from build123d import *

# Parameters (mm, degrees)
SKETCH2_W      = 150
SKETCH2_H      = 70
EXTRUDE1_DEPTH = 20
SKETCH3_W      = 20.4
SKETCH3_H      = 20.4
EXTRUDE2_DEPTH = 20
SKETCH6_W      = 20.4
SKETCH6_H      = 20.4
EXTRUDE5_DEPTH = 20
EXTRUDE6_DEPTH = 20


with BuildPart() as part:
    # Sketch2 → Extrude1 (new body)
    with BuildSketch(Plane(origin=(0, 0, 0), x_dir=(1, 0, 0), z_dir=(0, 1, 0))):
        Rectangle(SKETCH2_W, SKETCH2_H)
    extrude(amount=EXTRUDE1_DEPTH)

    # Sketch3 → Extrude2 (cut)
    with BuildSketch(Plane(origin=(0, 20, 0), x_dir=(1, 0, 0), z_dir=(0, 1, 0))):
        with Locations((0, 12.2)):
            Rectangle(SKETCH3_W, SKETCH3_H)
    extrude(amount=-EXTRUDE2_DEPTH, mode=Mode.SUBTRACT)

    # Sketch6 → Extrude5 (cut)
    with BuildSketch(Plane(origin=(0, 20, 0), x_dir=(1, 0, 0), z_dir=(0, 1, 0))):
        with Locations((-57.5, 4.8)):
            Rectangle(SKETCH6_W, SKETCH6_H)
        with Locations((57.5, 4.8)):
            Rectangle(SKETCH6_W, SKETCH6_H)
    extrude(amount=-EXTRUDE5_DEPTH, mode=Mode.SUBTRACT)

    # Sketch7 → Extrude6 (cut)
    with BuildSketch(Plane(origin=(0, 20, 0), x_dir=(1, 0, 0), z_dir=(0, 1, 0))):
        Polygon((-70.635231965, -35), (-75, -32.48), (-75, -35), align=None)
        Polygon((-75, 35), (-70.635231965, 35), (-75, 32.48), align=None)
        Polygon((75, -35), (70.635231965, -35), (75, -32.48), align=None)
        Polygon((70.635231965, 35), (75, 32.48), (75, 35), align=None)
    extrude(amount=-EXTRUDE6_DEPTH, mode=Mode.SUBTRACT)


solid = part.part
CAD build for the part. Positions are in the model's coordinates, mm. A direction names the side the tool comes from. Give positions to 0.01 mm unless a question says otherwise; leave off trailing zeros. Write each loop counter-clockwise with the first axis right and the second up, starting at its lowest first coordinate (ties: lowest second). Pieces come first, ordered by that corner, then holes. Notation, with made-up numbers: (43, -22.75) - (61, -22.75) arc R19 ccw to (61, -1.75) - close; hole circle Ø1 at (46, 1.25). An arc over 180 degrees is marked (long way). Answer as CSV lines item,"result".
Q1. Drill centre lines: line 1 (X direction, y = 18, z = -6); line 2 (Z direction, x = 58.5, y = 5.75); line 3 (Z direction, x = 7, y = 13.25). Where is each one in solid material? Low to high. Write a range as from..to.
Result set:
line 1,"-75..-67.7, -47.3..-10.2, 10.2..47.3, 67.7..75"
line 2,"-35..-15, 5.4..35"
line 3,"-35..-22.4, -2..35"
Q2. Band-saw the part on B-B (y = 5.25). Give the cut face in (x, z), and give its area (3 significant figures).
Result set:
outline,"(-75, -32.48) - (-70.64, -35) - (70.64, -35) - (75, -32.48) - (75, 32.48) - (70.64, 35) - (-70.64, 35) - (-75, 32.48) - close; hole (-67.7, -15) - (-47.3, -15) - (-47.3, 5.4) - (-67.7, 5.4) - close; hole (-10.2, -22.4) - (10.2, -22.4) - (10.2, -2) - (-10.2, -2) - close; hole (47.3, -15) - (67.7, -15) - (67.7, 5.4) - (47.3, 5.4) - close"
area,"9,230 mm²"
Q3. Pull direction Z, two halves, no side cores. Call faces 1 (the face through (-1, 20, 0)), 2 (the face through (57, 10, -15)), 3 (the face through (47.3, 10, -5)), 4 (the face through (-72.787, 10.14, 33.758)): released by +Z, released by -Z, zero draft, split by the parting line, or undercut.
Result set:
face 1,"zero draft"
face 2,"undercut"
face 3,"undercut"
face 4,"released by +Z"
Q4. 3-axis set-ups, long thin cutter, end or side, ignore diameter. For faces 5 (the face through (-47.3, 10, -5)), 6 (the face through (-1, 0, 0)): which of +Z, -Z, +X, -X, +Y, -Y reach the whole face in a straight line?
Result set:
face 5,"+Y, -Y"
face 6,"+Z, -Z, +X, -X, -Y"
Q5. Band-saw the part on A-A (x = 61). Give the cut face in (y, z), and give its area (3 significant figures).
Result set:
outline,"(0, -35) - (20, -35) - (20, -15) - (0, -15) - close; (0, 5.4) - (20, 5.4) - (20, 35) - (0, 35) - close"
area,"992 mm²"
Q6. Band-saw the part on C-C (z = -12). Give the cut face in (x, y).
Result set:
outline,"(-75, 0) - (-67.7, 0) - (-67.7, 20) - (-75, 20) - close; (-47.3, 0) - (-10.2, 0) - (-10.2, 20) - (-47.3, 20) - close; (10.2, 0) - (47.3, 0) - (47.3, 20) - (10.2, 20) - close; (67.7, 0) - (75, 0) - (75, 20) - (67.7, 20) - close"
